The drawing under review shows one solid part. Ordinate dimensions are in mm from its lowest x, y, z. Give positions to 0.01 mm unless a question says otherwise; leave off trailing zeros. Order: outer loops, then holes, each group sorted by start corner. A loop starts at its lowest first (then second) coordinate and runs counter-clockwise, first axis right, second up. Notation, with made-up numbers: (37, 87) - (93, 87) arc R13 cw to (93, 92) - close; hole circle Ø8 at (-30.5, -27). An arc over 180 degrees is marked (long way). Use CSV: the item, a comma, the result in double quotes.
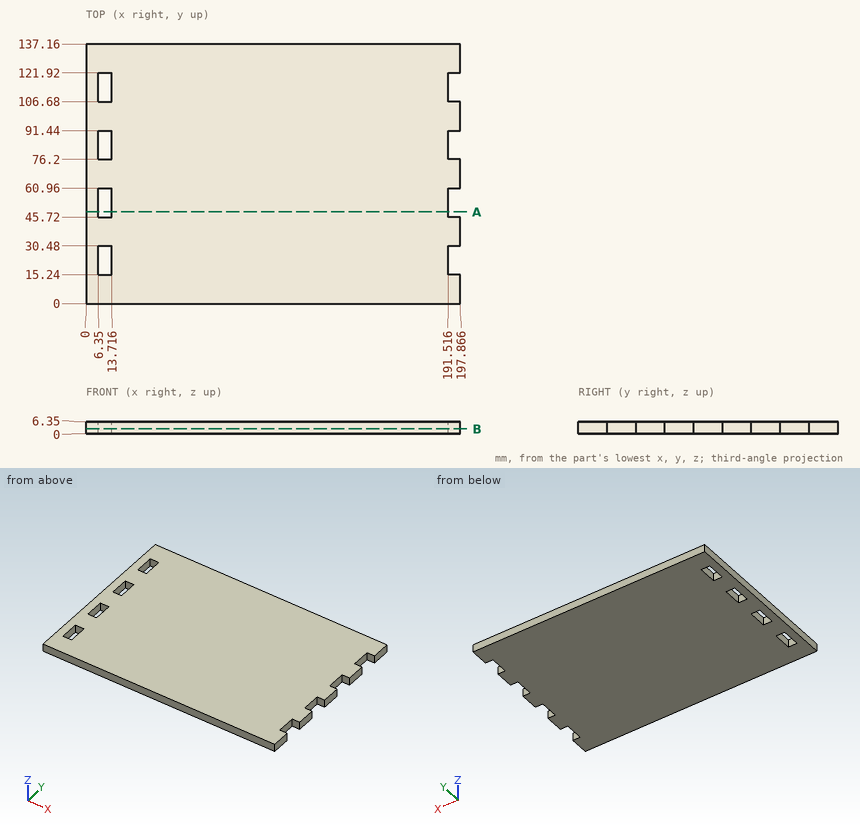
Item 1: Clearance check with a flat-ended pin moving along its axis: pin 1 (3 mm diameter, centred on y = 85.5, z = 4, fed in from +X). State where the tip first meets the part, or that it passes through.
Results list:
pin 1,"stops at x = 191.52"
Item 2: Take a section at B-B, the plane z = 2.5. State how many separate pieces and enclosed holes the cut face has, and give its area (3 significant figures).
Results list:
separate pieces,"1"
enclosed holes,"4"
area,"26,300 mm2"
Item 3: Take a section at A-A, the plane y = 48.5. Give the boundary of the cut face in (x, z).
Results list:
outline,"(0, 0) - (6.35, 0) - (6.35, 6.35) - (0, 6.35) - close; (13.72, 0) - (191.52, 0) - (191.52, 6.35) - (13.72, 6.35) - close"
Item 4: Wall thickness on L1, parallel to Y at x = 9.5, z = 5.5; L2, parallel to X at y = 59.5, z = 2.75: over which ranges is each line inside the solid? List them lowest first.
Results list:
L1,"y = 0 to 15.24, 30.48 to 45.72, 60.96 to 76.2, 91.44 to 106.68, 121.92 to 137.16"
L2,"x = 0 to 6.35, 13.72 to 191.52"
